```python
from build123d import *

# Parameters (mm, degrees)
SKETCH1_R                       = 2.5
BOSS_EXTRUDE1_DEPTH             = 15
SKETCH2_R                       = 1
CUT_EXTRUDE1_DEPTH              = 16.411035007
TAP_DRILL_FOR_M4X0_7_TAP1_D     = 3.3
TAP_DRILL_FOR_M4X0_7_TAP1_DEPTH = 9
TAP_DRILL_FOR_M4X0_7_TAP1_TIP   = 0.991420021
SKETCH5_W                       = 3
SKETCH5_H                       = 1.793791595
SKETCH5_H_2                     = 1.526677924
CHAMFER1_SIZE                   = 0.5
CHAMFER1_SIZE2                  = 0.866025404
CHAMFER2_SIZE                   = 1.21
CHAMFER2_SIZE2                  = 0.698593826


with BuildPart() as part:
    # Sketch1 → Boss-Extrude1 (new body)
    with BuildSketch(Plane.XY):
        Circle(SKETCH1_R)
    extrude(amount=BOSS_EXTRUDE1_DEPTH)

    # Sketch2 → Cut-Extrude1 (cut, through all)
    with BuildSketch(Plane(origin=(0, 0, 0), x_dir=(-1, 0, 0), z_dir=(0, 0, -1))):
        Circle(SKETCH2_R)
    extrude(amount=-CUT_EXTRUDE1_DEPTH, mode=Mode.SUBTRACT)

    # Tap Drill for M4x0.7 Tap1
    with Locations(Plane(origin=(0, 0, 0), x_dir=(-1, 0, 0), z_dir=(0, 0, -1))):
        with Locations((0, 0)):
            Hole(TAP_DRILL_FOR_M4X0_7_TAP1_D / 2, depth=TAP_DRILL_FOR_M4X0_7_TAP1_DEPTH)
            with Locations((0, 0, -(TAP_DRILL_FOR_M4X0_7_TAP1_DEPTH + TAP_DRILL_FOR_M4X0_7_TAP1_TIP / 2))):  # 118° drill point
                Cone(0, TAP_DRILL_FOR_M4X0_7_TAP1_D / 2, TAP_DRILL_FOR_M4X0_7_TAP1_TIP, mode=Mode.SUBTRACT)

    # Sketch5 → Cut-Revolve1 (revolve, cut)
    with BuildSketch(Plane(origin=(0, 0, 0), x_dir=(0, 0, -1), z_dir=(1, 0, 0)), mode=Mode.PRIVATE) as cut_revolve1_sk:
        with Locations((-12.5, 2.896895798)):
            Rectangle(SKETCH5_W, SKETCH5_H)
        with Locations((-2.810109468, 3.163338962)):
            Rectangle(SKETCH5_W, SKETCH5_H_2)
    revolve(cut_revolve1_sk.sketch.rotate(Axis((0, 0, 0), (0, 0, 1)), 90), axis=Axis((0, 0, 0), (0, 0, 1)), mode=Mode.SUBTRACT)

    # Chamfer1
    chamfer1_edges = [part.edges().sort_by_distance(p)[0] for p in [
        (-1.65, 0, 0),
    ]]
    chamfer1_side = [part.faces().sort_by_distance(p)[0] for p in [
        (-2.429289322, 0, 0),
    ]]
    chamfer(chamfer1_edges, length=CHAMFER1_SIZE, length2=CHAMFER1_SIZE2, reference=chamfer1_side[0])

    # Chamfer2
    chamfer2_edges = [part.edges().sort_by_distance(p)[0] for p in [
        (1, 0, 15),
    ]]
    chamfer2_side = [part.faces().sort_by_distance(p)[0] for p in [
        (1, 0, 12.195279701),
    ]]
    chamfer(chamfer2_edges, length=CHAMFER2_SIZE, length2=CHAMFER2_SIZE2, reference=chamfer2_side[0])


solid = part.part
```
Geometry: final body of the model. Coordinates: model frame, mm. A direction names the side the tool comes from. Give positions to 0.01 mm unless a question says otherwise; leave off trailing zeros. Order: outer loops, then holes, each group sorted by start corner. A loop starts at its lowest first (then second) coordinate and runs counter-clockwise, first axis right, second up. Notation, with made-up numbers: M -12,-12.75 L 43,-12.75 A10 cw 43,5.25 Z; hole C 71.25,5.5 d5. An arc over 180 degrees is marked long. Answer as CSV lines item,"result". Start each with the question number.
1) Cut plane C-C (z = 12). Output: boundary loops of the cut face in (x, y), then the cut area to 3 significant figures.
2) Mould query, pull axis Y, two halves, no side actions, for faces 3 (the flat face through (-1, -2, 14)), 4 (the cylindrical face through (1.474, -1.352, 12.479)), 5 (the cylindrical face through (-1.216, 1.115, 4.99)), 6 (the cylindrical face through (0, -1, 12)). Classes: +Y half, -Y half, draft (parallel to the pull), parting line (faces both ways), or undercut.
3) Line query: line 1 (X direction, y = 0, z = 4.75); line 2 (X direction, y = 0, z = 10.35). Output: solid intervals per line, ascending. Write a range as from..to.
4) Set-up query: faces 1 (the cylindrical face through (-0.54, -2.44, 0.65)), 2 (the cylindrical face through (-1.29, -2.024, 2.789)). Return all of +Z, -Z, +X, -X, +Y, -Y with unobstructed straight access to the full face (end or side cutting, diameter ignored); none if empty.
5) First-contact query: P1, Ø1.5, axis at x = -1, y = 0, coming from the -Z side; P2, Ø1, axis at x = -0.5, y = -1.5, coming from the +Z side; P3, Ø1.2, axis at x = 0, y = 0, coming from the -Z side. Flat tips, straight axial feed; report the tip coordinate or a pass-through.
Findings below:
1,outline,"C 0,0 d4; hole C 0,0 d2"
1,area,"9.42 mm²"
2,face 3,"draft"
2,face 4,"parting line"
2,face 5,"undercut"
2,face 6,"undercut"
3,line 1,"x = -2.5..-1.65, 1.65..2.5"
3,line 2,"x = -2.5..-1, 1..2.5"
4,face 1,"+Z, -Z"
4,face 2,"none"
5,P1,"stops at z = 0.69"
5,P2,"stops at z = 15"
5,P3,"passes through"
